Autodesk Fusion 360 part; units mm, degrees
sketch "草图1" plane through (0, 0, 0) normal (0, 0, 1) x (1, 0, 0)
  line L0 (-46.0977, 30) -> (46.0977, 30)
  line L1 (-46.0977, -30) -> (46.0977, -30)
  line L2 (-130, 0) -> (170, 0) construction
  line L3 (0, 120) -> (0, -120) construction
  circle A0 centre (-35, 17.5) radius 4
  circle A1 centre (35, 17.5) radius 4
  circle A2 centre (35, -17.5) radius 4
  circle A3 centre (-35, -17.5) radius 4
  arc A4 (46.0977, -30) -> (46.0977, 30) centre (0, 0) ccw
  arc A5 (-46.0977, 30) -> (-46.0977, -30) centre (0, 0) ccw
  dimension "d1" = 110
  dimension "d2" = 60
  dimension "d3" = 8
  dimension "d4" = 35
  dimension "d5" = 70
extrude "拉伸1" add sketch "草图1" against normal blind 10 makes body 1
sketch "草图2" plane through (0, -30, 0) normal (0, -1, 0) x (1, 0, 0)
  line L0 (46.0977, 0) -> (-46.0977, 0)
  line L1 (-46.0977, 0) -> (-46.0977, -10)
  line L2 (-46.0977, -10) -> (46.0977, -10)
  line L3 (46.0977, -10) -> (46.0977, 0)
  line L4 (-46.0977, 0) -> (46.0977, 0)
  line L5 (46.0977, 0) -> (46.0977, -10)
  line L6 (46.0977, -10) -> (-46.0977, -10)
  line L7 (-46.0977, -10) -> (-46.0977, 0)
  line L8 (-20, -7) -> (20, -7)
  line L9 (20, -7) -> (20, -10)
  line L10 (20, -10) -> (-20, -10)
  line L11 (-20, -10) -> (-20, -7)
  line L12 (0, 5) -> (0, -26.915) construction
  dimension "d8" = 40
  dimension "d9" = 3
extrude "拉伸2" cut sketch "草图2" against normal blind 80 contours L2 L6 L8 L9 L10 L11 bodies 1
sketch "草图3" plane through (0, 0, 0) normal (0, 0, 1) x (-1, 0, 0)
  circle A0 centre (35, 17.5) radius 4
  circle A1 centre (-35, -17.5) radius 4
  circle A2 centre (35, -17.5) radius 4
  circle A3 centre (-35, 17.5) radius 4
  arc A4 (46.0977, -30) -> (46.0977, 30) centre (0, 0) ccw
  line L0 (46.0977, 30) -> (-46.0977, 30)
  arc A5 (-46.0977, 30) -> (-46.0977, -30) centre (0, 0) ccw
  line L1 (-46.0977, -30) -> (46.0977, -30)
  circle A6 centre (0, 0) radius 25
  circle A7 centre (0, 0) radius 18
  dimension "d12" = 50
  dimension "d13" = 36
extrude "拉伸3" cut sketch "草图3" against normal blind 45 contours A7 bodies 1
extrude "拉伸4" add sketch "草图3" along normal blind 65 contours A6 bodies 1
sketch "草图4" plane through (0, 0, 0) normal (0, 1, 0) x (1, 0, 0)
  circle A0 centre (0, -35) radius 20
  circle A1 centre (0, -35) radius 15
  line L0 (-25, -65) -> (25, -65)
  dimension "d18" = 40
  dimension "d19" = 30
  dimension "d20" = 30
extrude "拉伸5" add sketch "草图4" against normal blind 38 bodies 1
extrude "拉伸6" cut sketch "草图4" against normal blind 60 contours A1 bodies 1
sketch "草图5" plane through (0, 0, 0) normal (0, 1, 0) x (1, 0, 0)
  line L0 (50, 0) -> (19.69, -65)
  line L1 (-19.69, -65) -> (-50, 0)
  line L2 (-19.69, -65) -> (-19.69, 0)
  line L3 (19.69, -65) -> (19.69, 0)
  line L4 (-60, 0) -> (-19.69, 0) construction
  line L5 (19.69, 0) -> (60, 0) construction
  line L6 (-50, 0) -> (-19.69, 0)
  line L7 (19.69, 0) -> (50, 0)
  dimension "d25" = 100
  dimension "d26" = 65
extrude "拉伸7" add sketch "草图5" along normal mid plane 10 separate body makes body 2 at (-29.7933, 5, 21.6667) makes body 3 at (29.7933, 5, 21.6667)
combine "合并1" operation add target body 1 tool bodies 3 2
Design review of the part built by this model. Coordinates are the model's own, in mm. A direction names the side the tool comes from. Give positions to 0.01 mm unless a question says otherwise; leave off trailing zeros. Loops run counter-clockwise (first coordinate to the right, second up) from the corner with the lowest first, then second, coordinate; pieces in that order, holes last. Notation, with made-up numbers: (82, -11.5) - (131, -11.5) arc R30 cw to (131, 13.5) - close; hole circle Ø5 at (39, 1). An arc over 180 degrees is marked (long way). Use CSV: the item, a comma, the result in double quotes. Start each with the question number.
1. Machinability: for faces 5 (the flat face through (-32, 5, 21)), 6 (the flat face through (34, 5, 21)), 7 (the flat face through (-32, -5, 21)), which of the approach directions +Z, -Z, +X, -X, +Y, -Y give a long, thin tool a straight path to every point of the face, cutting with its end or side? Answer none if there is none.
2. Add section A-A (x = 0). State the section outline as (y, z) points, plus the area to 3 significant figures.
3. Add section D-D (x = 35). State the section outline as (y, z) points, plus the area to 3 significant figures.
4. Insertion check: P1, Ø13, axis at x = -36.5, z = 19, coming from the +Y side; P2, Ø3, axis at x = 7, z = -6, coming from the -Y side; P3, Ø13, axis at x = 35, y = 17.5, coming from the +Z side. Each pin has a flat end and moves straight along its axis. Give the tip position at first contact, or say it passes through.
5. Add section B-B (z = -2.5). State the section outline as (x, y) points.
6. Draft analysis for pull direction Z (two halves, no side actions). For faces 1 (the cylindrical face through (-19.98, -28.89, 34.12)), 2 (the cylindrical face through (-1.953, -18.734, 20.128)), 3 (the flat face through (-37.07, -0.07, 27.73)), 4 (the flat face through (-1, 30, -4)), state which applies: released by +Z, released by -Z, zero draft, split by the parting line, or undercut.
7. Wall thickness on L1, parallel to Y at x = 35, z = -7.25; L2, parallel to Z at x = 0, y = -23; L3, parallel to Z at x = 0, y = -14: over which ranges is each line inside the solid? List them lowest first.
8. Add section C-C (y = 9). State the section outline as (x, z) points.
Results found:
1,face 5,"+Z, -X, +Y"
1,face 6,"+Z, +X, +Y"
1,face 7,"+Z, -X, -Y"
2,outline,"(-38, 15) - (-25, 15) - (-25, 0) - (-30, 0) - (-30, -7) - (-18, -7) - (-18, 15) - (0, 15) - (0, 20) - (-38, 20) - close; (-38, 50) - (0, 50) - (0, 55) - (-18, 55) - (-18, 65) - (-25, 65) - (-25, 55) - (-38, 55) - close; (18, -7) - (30, -7) - (30, 0) - (25, 0) - (25, 65) - (18, 65) - close"
2,area,"1,180 mm²"
3,outline,"(-30, -10) - (-21.5, -10) - (-21.5, 0) - (-30, 0) - close; (-13.5, -10) - (13.5, -10) - (13.5, 0) - (5, 0) - (5, 32.17) - (-5, 32.17) - (-5, 0) - (-13.5, 0) - close; (21.5, -10) - (30, -10) - (30, 0) - (21.5, 0) - close"
3,area,"762 mm²"
4,P1,"stops at y = 5"
4,P2,"stops at y = -30"
4,P3,"stops at z = 0"
5,outline,"(-46.1, -30) - (46.1, -30) arc R55 ccw to (46.1, 30) - (-46.1, 30) arc R55 ccw to start; hole circle Ø8 at (-35, -17.5); hole circle Ø8 at (-35, 17.5); hole circle Ø36 at (0, 0); hole circle Ø8 at (35, -17.5); hole circle Ø8 at (35, 17.5)"
6,face 1,"undercut"
6,face 2,"undercut"
6,face 3,"released by +Z"
6,face 4,"zero draft"
7,L1,"y = -30 to -21.5, -13.5 to 13.5, 21.5 to 30"
7,L2,"z = -7 to 20, 50 to 65"
7,L3,"z = 15 to 20, 50 to 55"
8,outline,"(-54.26, -10) - (-20, -10) - (-20, -7) - (-15.59, -7) - (-15.59, 65) - (-23.32, 65) - (-23.32, 0) - (-54.26, 0) - close; (15.59, -7) - (20, -7) - (20, -10) - (54.26, -10) - (54.26, 0) - (23.32, 0) - (23.32, 65) - (15.59, 65) - close"
